Geometry: see drawing. Coordinates: mm, zero at the bounding-box minimum. A direction names the side the tool comes from. Coordinates: 2 decimals unless noted, no trailing zeros. Loops run counter-clockwise (first coordinate to the right, second up) from the corner with the lowest first, then second, coordinate; pieces in that order, holes last.
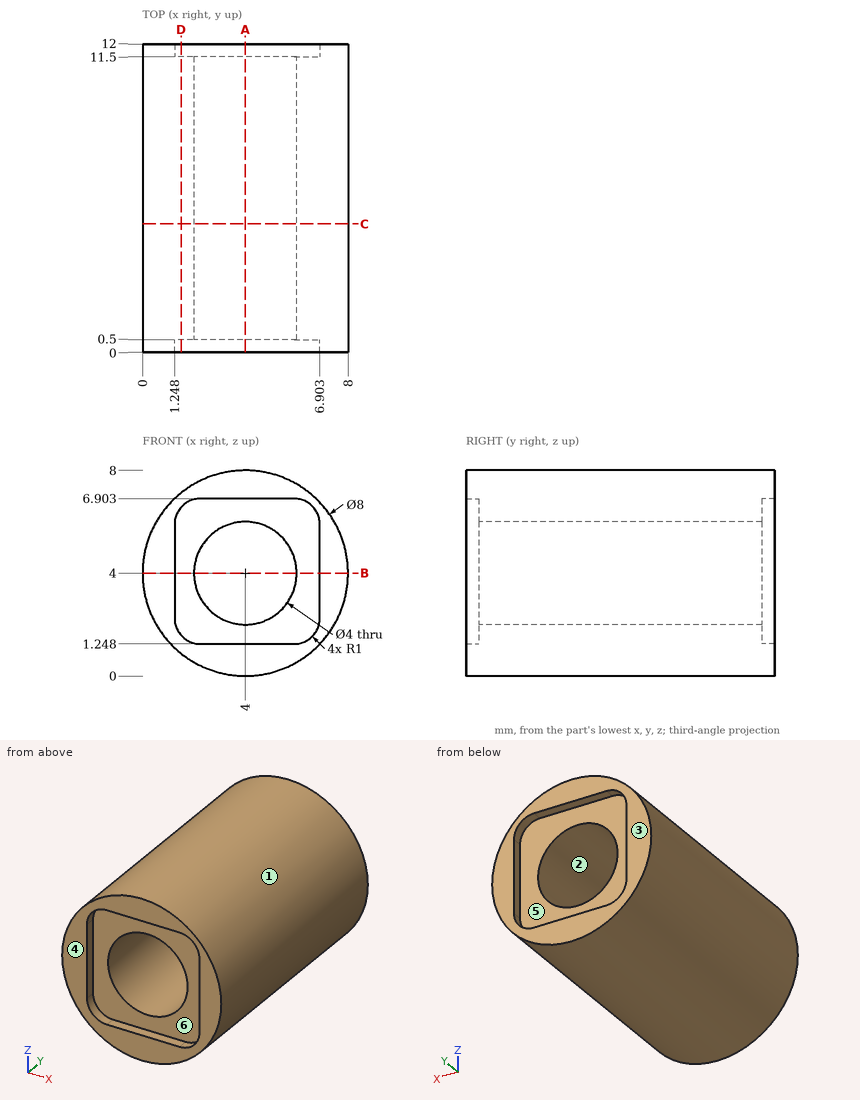
Item 1: Section query B-B (z = 4). Output: boundary loops of the cut face in (x, y).
Result:
outline: (0, 0) - (1.25, 0) - (1.25, 0.5) - (2, 0.5) - (2, 11.5) - (1.25, 11.5) - (1.25, 12) - (0, 12) - close; (6, 0.5) - (6.9, 0.5) - (6.9, 0) - (8, 0) - (8, 12) - (6.9, 12) - (6.9, 11.5) - (6, 11.5) - close
Item 2: Section query C-C (y = 5). Output: boundary loops of the cut face in (x, z), then the cut area to 3 significant figures.
Result:
outline: circle Ø8 at (4, 4); hole circle Ø4 at (4, 4)
area: 37.7 mm2
Item 3: Reachability of the marked faces 4, 5 and 6 from +Z, -Z, +X, -X, +Y, -Y: full face, straight path, thin tool, end or side. Return the list, or none.
Result:
face 4: +Z, -Z, +X, -X, -Y
face 5: +Y
face 6: -Y
Item 4: Section query D-D (x = 1.5). Output: boundary loops of the cut face in (y, z).
Result:
outline: (0, 0.88) - (12, 0.88) - (12, 1.58) - (11.5, 1.58) - (11.5, 6.57) - (12, 6.57) - (12, 7.12) - (0, 7.12) - (0, 6.57) - (0.5, 6.57) - (0.5, 1.58) - (0, 1.58) - close
Item 5: Section query A-A (x = 4). Output: boundary loops of the cut face in (y, z).
Result:
outline: (0, 0) - (12, 0) - (12, 1.25) - (11.5, 1.25) - (11.5, 2) - (0.5, 2) - (0.5, 1.25) - (0, 1.25) - close; (0, 6.9) - (0.5, 6.9) - (0.5, 6) - (11.5, 6) - (11.5, 6.9) - (12, 6.9) - (12, 8) - (0, 8) - close
Item 6: Contact query for flat-ended pins moving along their axis: P1, Ø0.6, axis at y = 0.5, z = 3, coming from the +X side; P2, Ø2, axis at x = 2.5, y = 3.5, coming from the -Z side; P3, Ø1, axis at x = 3, y = 7, coming from the +Z side; P4, Ø3, axis at x = 1.5, z = 7, coming from the -Y side. Output: stop coordinate, or through.
Result:
P1: stops at x = 7.94
P2: stops at z = 0.03
P3: stops at z = 7.97
P4: stops at y = 0
Item 7: Line query: L1, parallel to Z at x = 4, y = 5.75; L2, parallel to Y at x = 2, z = 6.5; L3, parallel to Z at x = 5.5, y = 9.75 (1 decimal). Output: solid intervals per line, ascending.
Result:
L1: z = 0 to 2, 6 to 8
L2: y = 0.5 to 11.5
L3: z = 0.3 to 2.7, 5.3 to 7.7
Item 8: Mould query, pull axis X, two halves, no side actions, for the marked faces 1, 2 and 3. Classes: +X half, -X half, draft (parallel to the pull), parting line (faces both ways), or undercut.
Result:
face 1: parting line
face 2: undercut
face 3: draft
